Design review of the part built by this model. Coordinates are the model's own, in mm. Face numbers are marked on the shaded views. A direction names the side the tool comes from. Coordinates: 2 decimals unless noted, no trailing zeros. Write each loop counter-clockwise with the first axis right and the second up, starting at its lowest first coordinate (ties: lowest second). Pieces come first, ordered by that corner, then holes.
Q1. For pin 1 Ø4 at (x, y) = (13.42, -7.75) entering from -Z; pin 2 Ø0.5 at (y, z) = (0, 1) entering from -X; pin 3 Ø1 at (y, z) = (-2.5, 18) entering from +X, all flat-tipped, find the tip position at first contact; note any pin that passes through.
Q2. The part is to be moulded in two halves that separate along Z. For the marked faces 6, 7 and 8, say which applies: released by +Z, released by -Z, zero draft, split by the parting line, or undercut.
Q3. Take a section at B-B, the plane y = -15.5. Write out the cut boundary in (x, z).
Q4. Take a section at A-A, the plane z = 4.25. Write out the cut boundary in (x, y).
Q5. For L1, parallel to Y at x = 0, z = 24.05; L2, parallel to Y at x = 12.5, z = 21.75; L3, parallel to X at y = -7.75, z = 23.45, list the stretches that pass through material, from the lowest coordinate up.
Q6. For the marked faces 1, 2, 3, 4 and 5, list the 3-axis set-ups (+Z, -Z, +X, -X, +Y, -Y) from which the entire face can be reached by the end or side of a thin tool; tool diameter is ignored.
Q7. Take a section at D-D, the plane z = 22.25. Write out the cut boundary in (x, y).
Q8. Take a section at C-C, the plane x = 0. State how many separate pieces and enclosed holes the cut face has, plus the area to 3 significant figures.
from build123d import *

# Parameters (mm, degrees)
BOSS_EXTRUDE1_DEPTH                                  = 10
F_5_0MM_DOWEL_HOLE1_D                                = 5
F_5_0MM_DOWEL_HOLE1_CSINK_D                          = 5.05
F_5_0MM_DOWEL_HOLE1_CSINK_ANGLE                      = 90
SKETCH5_R                                            = 10
BOSS_EXTRUDE2_DEPTH                                  = 10
SKETCH6_R                                            = 11.5
BOSS_EXTRUDE3_DEPTH                                  = 1
SKETCH7_R                                            = 20
BOSS_EXTRUDE4_DEPTH                                  = 4
CSK_FOR_M3_HEX_SOCKET_COUNTERSUNK_HEAD_S_D           = 3.4
CSK_FOR_M3_HEX_SOCKET_COUNTERSUNK_HEAD_S_CSINK_D     = 6.94
CSK_FOR_M3_HEX_SOCKET_COUNTERSUNK_HEAD_S_CSINK_ANGLE = 90
F_13_0_13_DIAMETER_HOLE1_D                           = 13
SKETCH12_R                                           = 10
CUT_EXTRUDE1_DEPTH                                   = 0.2
CUT_EXTRUDE2_START                                   = -10.2
CUT_EXTRUDE2_DEPTH                                   = 10.2
CHAMFER1_SIZE                                        = 0.5


with BuildPart() as part:
    # Sketch1 → Boss-Extrude1 (new body)
    with BuildSketch(Plane.XY):
        Polygon((-4.907477288, 8.5), (-9.814954576, 0), (-4.907477288, -8.5), (4.907477288, -8.5), (9.814954576, 0), (4.907477288, 8.5), align=None)
    extrude(amount=BOSS_EXTRUDE1_DEPTH)

    # Ø5.0mm Dowel Hole1 (through all)
    with Locations(Plane(origin=(0, 8.5, 0), x_dir=(1, 0, 0), z_dir=(0, 1, 0))):
        with Locations((-9.814954576, -5), (9.814954576, -5)):
            CounterSinkHole(F_5_0MM_DOWEL_HOLE1_D / 2, F_5_0MM_DOWEL_HOLE1_CSINK_D / 2, counter_sink_angle=F_5_0MM_DOWEL_HOLE1_CSINK_ANGLE)

    # Sketch5 → Boss-Extrude2 (add)
    with BuildSketch(Plane.XY.offset(10)):
        Circle(SKETCH5_R)
    extrude(amount=BOSS_EXTRUDE2_DEPTH)

    # Sketch6 → Boss-Extrude3 (add)
    with BuildSketch(Plane.XY.offset(20)):
        Circle(SKETCH6_R)
    extrude(amount=BOSS_EXTRUDE3_DEPTH)

    # Sketch7 → Boss-Extrude4 (add)
    with BuildSketch(Plane.XY.offset(21)):
        Circle(SKETCH7_R)
    extrude(amount=BOSS_EXTRUDE4_DEPTH)

    # CSK for M3 Hex Socket Countersunk Head Screw1 (through all)
    with Locations(Plane(origin=(0, 0, 21), x_dir=(-1, 0, 0), z_dir=(0, 0, -1))):
        with Locations((0, 15.5), (13.423393759, 7.75), (13.423393759, -7.75), (0, -15.5), (-13.423393759, -7.75), (-13.423393759, 7.75)):
            CounterSinkHole(CSK_FOR_M3_HEX_SOCKET_COUNTERSUNK_HEAD_S_D / 2, CSK_FOR_M3_HEX_SOCKET_COUNTERSUNK_HEAD_S_CSINK_D / 2, counter_sink_angle=CSK_FOR_M3_HEX_SOCKET_COUNTERSUNK_HEAD_S_CSINK_ANGLE)

    # Ø13.0 (13) Diameter Hole1 (through all)
    with Locations(Plane.XY.offset(25)):
        with Locations((0, 0)):
            Hole(F_13_0_13_DIAMETER_HOLE1_D / 2)

    # Sketch12 → Cut-Extrude1 (cut)
    with BuildSketch(Plane(origin=(0, 0, 10), x_dir=(-1, 0, 0), z_dir=(0, 0, -1))):
        Circle(SKETCH12_R)
        Polygon((4.907477288, 8.5), (-4.907477288, 8.5), (-9.814954576, 0), (-4.907477288, -8.5), (4.907477288, -8.5), (9.814954576, 0), align=None, mode=Mode.SUBTRACT)
    extrude(amount=-CUT_EXTRUDE1_DEPTH, mode=Mode.SUBTRACT)

    # Sketch13 → Cut-Extrude2 (cut)
    with BuildSketch(Plane(origin=(0, 0, 0), x_dir=(-1, 0, 0), z_dir=(0, 0, -1)).offset(CUT_EXTRUDE2_START)):
        Polygon((-5.222431864, 7.954482672), (-4.277568136, 8.5), (-4.907477288, 8.5), align=None)
        Polygon((4.907477288, 8.5), (4.277568136, 8.5), (5.222431864, 7.954482672), align=None)
        Polygon((-9.5, -0.545517328), (-9.5, 0.545517328), (-9.814954576, 0), align=None)
        Polygon((9.814954576, 0), (9.5, 0.545517328), (9.5, -0.545517328), align=None)
        Polygon((-4.277568136, -8.5), (-5.222431864, -7.954482672), (-4.907477288, -8.5), align=None)
        Polygon((4.907477288, -8.5), (5.222431864, -7.954482672), (4.277568136, -8.5), align=None)
    extrude(amount=CUT_EXTRUDE2_DEPTH, mode=Mode.SUBTRACT)

    # Chamfer1
    chamfer1_edges = [part.edges().sort_by_distance(p)[0] for p in [
        (6.5, 0, 0),
        (0, 8.5, 0),
        (7.361215932, 4.25, 0),
        (7.361215932, -4.25, 0),
        (0, -8.5, 0),
        (-7.361215932, -4.25, 0),
        (-7.361215932, 4.25, 0),
        (9.5, 0, 0),
        (4.75, -8.227241336, 0),
        (-4.75, -8.227241336, 0),
        (-9.5, 0, 0),
        (-4.75, 8.227241336, 0),
        (4.75, 8.227241336, 0),
    ]]
    chamfer(chamfer1_edges, length=CHAMFER1_SIZE)


solid = part.part
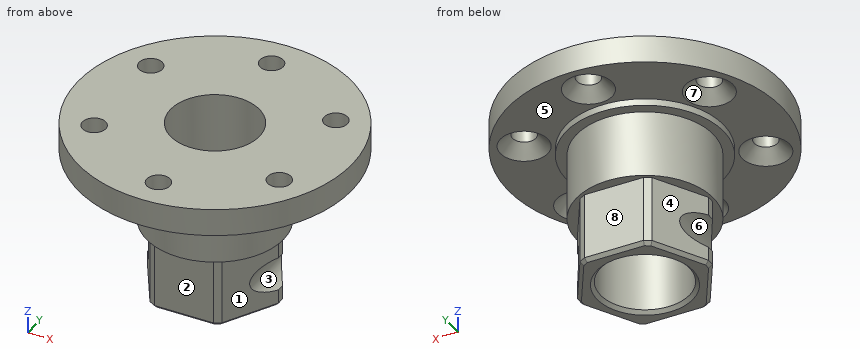
Responses:
1. pin 1: stops at z = 22.47
1. pin 2: stops at x = -9.5
1. pin 3: stops at x = 9.8
2. face 6: undercut
2. face 7: released by -Z
2. face 8: zero draft
3. outline: (-12.64, 21) - (-3.47, 21) - (-1.7, 22.77) - (-1.7, 25) - (-12.64, 25) - close; (1.7, 22.77) - (3.47, 21) - (12.64, 21) - (12.64, 25) - (1.7, 25) - close
4. outline: (-7.43, -4.13) - (-5.22, -7.95) - (-4.28, -8.5) - (4.28, -8.5) - (5.22, -7.95) - (7.43, -4.13) - (7.43, 4.13) - (5.22, 7.95) - (4.28, 8.5) - (-4.28, 8.5) - (-5.22, 7.95) - (-7.43, 4.13) - close; hole circle Ø13 at (0, 0)
5. L1: y = -20 to -17.2, -13.8 to -6.5, 6.5 to 13.8, 17.2 to 20
5. L2: y = -15.61 to -10.31, -5.19 to 5.19, 10.31 to 15.61
5. L3: x = -18.44 to -15.12, -11.72 to 11.72, 15.12 to 18.44
6. face 1: -Z, +X, -Y
6. face 2: -Z, +X, -X, -Y
6. face 3: +X, +Y, -Y
6. face 4: -Z, -X, +Y
6. face 5: -Z
7. outline: circle Ø40 at (0, 0); hole circle Ø4.44 at (-13.42, -7.75); hole circle Ø4.44 at (-13.42, 7.75); hole circle Ø13 at (0, 0); hole circle Ø4.44 at (0, -15.5); hole circle Ø4.44 at (0, 15.5); hole circle Ø4.44 at (13.42, -7.75); hole circle Ø4.44 at (13.42, 7.75)
8. separate pieces: 4
8. enclosed holes: 0
8. area: 193 mm2
